The drawing under review shows one solid part. Ordinate dimensions are in mm from its lowest x, y, z. A direction names the side the tool comes from. Give positions to 0.01 mm unless a question says otherwise; leave off trailing zeros. Loops run counter-clockwise (first coordinate to the right, second up) from the corner with the lowest first, then second, coordinate; pieces in that order, holes last. Notation, with made-up numbers: (-21.75, 38) - (22.25, 38) arc R26 ccw to (22.25, 52) - close; hole circle Ø7 at (-3, -12). An arc over 180 degrees is marked (long way). Return JSON: item names as keys, results as strings. Group by question number.
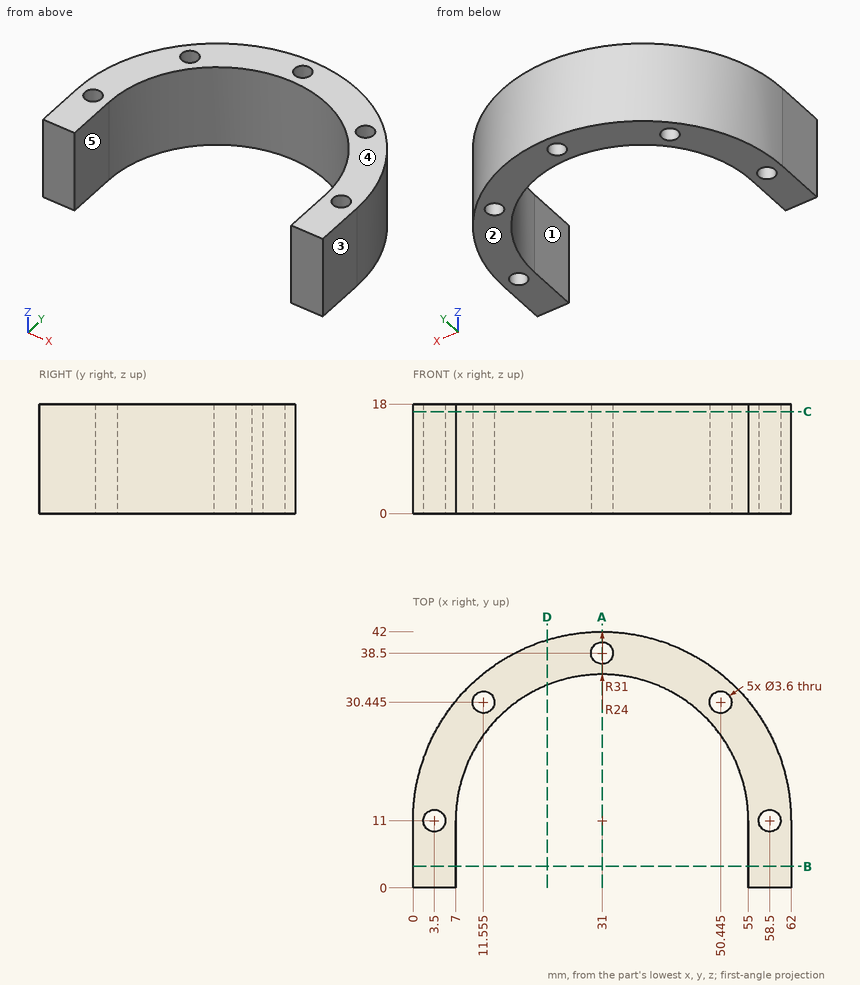
1) We need section A-A, the plane x = 31. Write out the cut boundary in (y, z).
2) We need section D-D, the plane x = 22. Write out the cut boundary in (y, z) (1 decimal).
3) To check wall thickness, follow line 1 (X direction, y = 29.5, z = 16) (1 decimal); line 2 (Y direction, x = 31, z = 9.5); line 3 (X direction, y = 8, z = 11). State the ranges of each line that lie inside material, in increasing order.
4) We need section B-B, the plane y = 3.5. Write out the cut boundary in (x, z).
5) For pin 1 Ø10 at (y, z) = (15, 6) entering from +X; pin 2 Ø4 at (y, z) = (30.5, 12) entering from +X; pin 3 Ø8 at (x, z) = (20, 2) entering from -Y (1 decimal); pin 4 Ø1.5 at (x, z) = (8, 5.5) entering from +Y (1 decimal), all flat-tipped, find the tip position at first contact; note any pin that passes through.
6) We need section C-C, the plane z = 16.75. Write out the cut boundary in (x, y) (1 decimal), plus the area to 3 significant figures.
7) Draft analysis for pull direction X (two halves, no side actions). For the marked faces 1, 2 and 3, state which applies: +X half, -X half, draft (parallel to the pull), parting line (faces both ways), or undercut.
8) Tool access review of the marked faces 4 and 5: name each direction out of +Z, -Z, +X, -X, +Y, -Y from which nothing blocks a thin tool from reaching the whole face with its end or side.
Findings:
{
 "1": {"outline": "(35, 0) - (36.7, 0) - (36.7, 18) - (35, 18) - close; (40.3, 0) - (42, 0) - (42, 18) - (40.3, 18) - close"},
 "2": {"outline": "(33.2, 0) - (40.7, 0) - (40.7, 18) - (33.2, 18) - close"},
 "3": {"line 1": "x = 6.1 to 10, 13.1 to 15.7, 46.3 to 48.9, 52 to 55.9", "line 2": "y = 35 to 36.7, 40.3 to 42", "line 3": "x = 0 to 7, 55 to 62"},
 "4": {"outline": "(0, 0) - (7, 0) - (7, 18) - (0, 18) - close; (55, 0) - (62, 0) - (62, 18) - (55, 18) - close"},
 "5": {"pin 1": "stops at x = 62", "pin 2": "stops at x = 56.59", "pin 3": "stops at y = 29.7", "pin 4": "stops at y = 32.6"},
 "6": {"outline": "(0, 0) - (7, 0) - (7, 11) arc R24 cw to (55, 11) - (55, 0) - (62, 0) - (62, 11) arc R31 ccw to (0, 11) - close; hole circle Ø3.6 at (3.5, 11); hole circle Ø3.6 at (11.6, 30.4); hole circle Ø3.6 at (31, 38.5); hole circle Ø3.6 at (50.4, 30.4); hole circle Ø3.6 at (58.5, 11)", "area": "708 mm^2"},
 "7": {"face 1": "undercut", "face 2": "draft", "face 3": "+X half"},
 "8": {"face 4": "+Z, +X, -X, +Y, -Y", "face 5": "+Z, -Z, -Y"}
}
